from build123d import *

# Parameters (mm, degrees)
F0_R          = 6.35
F1_DEPTH      = 33.02
F2_R          = 6.35
F3_R          = 0.79375
F4_DEPTH      = 6.351
F4_DEPTH_BACK = 25.4
F5_R          = 4.318
F6_DEPTH      = 19.05
F7_R          = 2.54


with BuildPart() as f1:
    # F0 (on Top) → F1 (new body)
    with BuildSketch(Plane.XY):
        Circle(F0_R)
    extrude(amount=F1_DEPTH)

    # F2
    f2_edges = [f1.edges().sort_by_distance(p)[0] for p in [
        (-6.35, 0, 33.02),
    ]]
    fillet(f2_edges, radius=F2_R)

    # F3 (on Right) → F4 (cut, two sides)
    with BuildSketch(Plane.YZ) as f4_sk:
        with Locations((0, 25.4)):
            Circle(F3_R)
    extrude(amount=F4_DEPTH, mode=Mode.SUBTRACT)
    extrude(f4_sk.sketch, amount=-F4_DEPTH_BACK, mode=Mode.SUBTRACT)

    # F5 (on face) → F6 (cut)
    with BuildSketch(Plane(origin=(0, 0, 0), x_dir=(1, 0, 0), z_dir=(0, 0, -1))):
        Circle(F5_R)
    extrude(amount=-F6_DEPTH, mode=Mode.SUBTRACT)

    # F7
    f7_edges = [f1.edges().sort_by_distance(p)[0] for p in [
        (-4.318, 0, 19.05),
    ]]
    fillet(f7_edges, radius=F7_R)


solid = f1.part
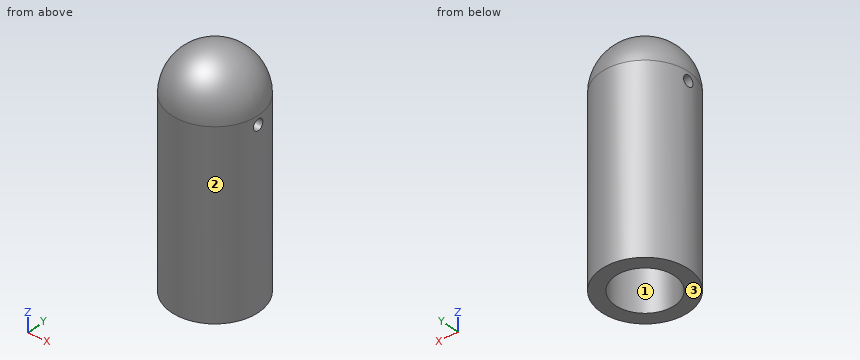
Source: CAD feature listing. Evaluate the final solid. Frame: model axes, mm. Face numbers are marked on the shaded views. Coordinates: 2 decimals unless noted, no trailing zeros. Loops run counter-clockwise (first coordinate to the right, second up) from the corner with the lowest first, then second, coordinate; pieces in that order, holes last. Notation, with made-up numbers: (-39, 29.5) -> (-6, 29.5) arc R20 cw to (-6, 66.5) -> close; hole circle Ø3 at (48.25, -23). An arc over 180 degrees is marked (long way). Answer in a Markdown table with one row per item. Add a question column.
Q1. Section B-B on x = 5. Return the cut outline in (y, z).
Q2. Contact query for flat-ended pins moving along their axis: pin 1 Ø1 at (y, z) = (-4.5, 21) entering from -X; pin 2 Ø2 at (x, z) = (4, 12) entering from -Y; pin 3 Ø5 at (x, z) = (2, 29) entering from -Y; pin 4 Ø1.4 at (y, z) = (0, 25.4) entering from +X. Output: stop coordinate, or through.
Q3. Pull-direction query (Y, two-part tool) for the marked faces 1, 2 and 3; classes: pulls with the +Y half, pulls with the -Y half, needs draft (parallel to the pull), parting line crosses it, or undercut.
Q4. Section D-D on y = -5.5. Return the cut outline in (x, z), and give its area (3 significant figures).
Q5. Section A-A on z = 6. Return the cut outline in (x, y).
Q6. Section C-C on z = 19.5. Return the cut outline in (x, y).
Q7. Ray query, line 1 along X through (y, z) = (0, 8.75); line 2 along X through (y, z) = (1, 1.5). Return the intervals inside material, ascending.
Computed values:
| question | item | result |
|---|---|---|
| 1 | outline | (-3.91, 0) -> (3.91, 0) -> (3.91, 26.67) arc R3.91 ccw to (-3.91, 26.67) -> close; hole circle Ø1.59 at (0, 25.4) |
| 2 | pin 1 | stops at x = -4.93 |
| 2 | pin 2 | stops at y = -5.6 |
| 2 | pin 3 | stops at y = -6.32 |
| 2 | pin 4 | passes through |
| 3 | face 1 | undercut |
| 3 | face 2 | parting line crosses it |
| 3 | face 3 | needs draft |
| 4 | outline | (-3.17, 0) -> (3.17, 0) -> (3.17, 26.67) arc R3.17 ccw to (-3.17, 26.67) -> close |
| 4 | area | 185 mm^2 |
| 5 | outline | circle Ø12.7 at (0, 0); hole circle Ø8.64 at (0, 0) |
| 6 | outline | circle Ø12.7 at (0, 0) |
| 7 | line 1 | x = -6.35 to -4.32, 4.32 to 6.35 |
| 7 | line 2 | x = -6.27 to -4.2, 4.2 to 6.27 |
